For this review, take the finished solid that the model builds, in its own axes (mm). A direction names the side the tool comes from. Coordinates: 2 decimals unless noted, no trailing zeros. Loops run counter-clockwise (first coordinate to the right, second up) from the corner with the lowest first, then second, coordinate; pieces in that order, holes last. Notation, with made-up numbers: M 61,75.5 L 95,75.5 A29 ccw 95,107.5 Z; hole C -40,70.25 d2. An arc over 180 degrees is marked long. Put each result on its own line as item: value.
```python
from build123d import *

# Parameters (mm, degrees)
SKETCH_W        = 66
SKETCH_H        = 60
PAD_DEPTH       = 2
FILLET_R        = 4
SKETCH001_R     = 1.75
POCKET_DEPTH    = 2.001
PAD001_DEPTH    = 2
POCKET001_DEPTH = 2
FILLET001_R     = 1
FILLET002_R     = 1
FILLET003_R     = 1
FILLET004_R     = 1


with BuildPart() as part:
    # Sketch → Pad (new body)
    with BuildSketch(Plane.XY):
        Rectangle(SKETCH_W, SKETCH_H)
    extrude(amount=PAD_DEPTH)

    # Fillet
    fillet_edges = [part.edges().sort_by_distance(p)[0] for p in [
        (-33, -30, 1),
        (33, -30, 1),
        (33, 30, 1),
        (-33, 30, 1),
    ]]
    fillet(fillet_edges, radius=FILLET_R)

    # Sketch001 (on Face5 of Fillet) → Pocket (cut, through all)
    with BuildSketch(Plane.XY.offset(2)):
        with Locations((-29, 26)):
            Circle(SKETCH001_R)
        with Locations((29, 26)):
            Circle(SKETCH001_R)
        with Locations((29, -26)):
            Circle(SKETCH001_R)
        with Locations((-29, -26)):
            Circle(SKETCH001_R)
    extrude(amount=-POCKET_DEPTH, mode=Mode.SUBTRACT)

    # Sketch002 (on Face5 of Pocket) → Pad001 (join)
    with BuildSketch(Plane.XY.offset(2)):
        with BuildLine():
            ThreePointArc((-29.8, 22.901613), (-26.737258, 23.737258), (-25.901613, 26.8))
            Line((-25.901613, 26.8), (25.901613, 26.8))
            ThreePointArc((25.901613, 26.8), (26.737258, 23.737258), (29.8, 22.901613))
            Line((29.8, 22.901613), (29.8, -22.901613))
            ThreePointArc((29.8, -22.901613), (26.737258, -23.737258), (25.901613, -26.8))
            Line((-25.901613, -26.8), (25.901613, -26.8))
            ThreePointArc((-25.901613, -26.8), (-26.737258, -23.737258), (-29.8, -22.901613))
            Line((-29.8, 22.901613), (-29.8, -22.901613))
        make_face()
    extrude(amount=PAD001_DEPTH)

    # Sketch003 (on Face23 of Pad001) → Pocket001 (cut)
    with BuildSketch(Plane.XY.offset(4)):
        with BuildLine():
            ThreePointArc((-26.6, 20.283358), (-24.615938, 21.615938), (-23.283358, 23.6))
            Line((23.283358, 23.6), (-23.283358, 23.6))
            ThreePointArc((23.283358, 23.6), (24.615938, 21.615938), (26.6, 20.283358))
            Line((26.6, -20.283358), (26.6, 20.283358))
            ThreePointArc((26.6, -20.283358), (24.615938, -21.615938), (23.283358, -23.6))
            Line((-23.283358, -23.6), (23.283358, -23.6))
            ThreePointArc((-23.283358, -23.6), (-24.615938, -21.615938), (-26.6, -20.283358))
            Line((-26.6, 20.283358), (-26.6, -20.283358))
        make_face()
    extrude(amount=-POCKET001_DEPTH, mode=Mode.SUBTRACT)

    # Fillet001
    fillet001_edges = [part.edges().sort_by_distance(p)[0] for p in [
        (-25.901613, 26.8, 3),
        (-29.8, 22.901613, 3),
        (-29.8, -22.901613, 3),
        (-25.901613, -26.8, 3),
        (25.901613, 26.8, 3),
        (29.8, 22.901613, 3),
        (29.8, -22.901613, 3),
        (25.901613, -26.8, 3),
    ]]
    fillet(fillet001_edges, radius=FILLET001_R)

    # Fillet002
    fillet002_edges = [part.edges().sort_by_distance(p)[0] for p in [
        (-26.6, 20.283358, 3),
        (-23.283358, 23.6, 3),
        (23.283358, 23.6, 3),
        (26.6, 20.283358, 3),
        (26.6, -20.283358, 3),
        (23.283358, -23.6, 3),
        (-26.6, -20.283358, 3),
        (-23.283358, -23.6, 3),
    ]]
    fillet(fillet002_edges, radius=FILLET002_R)

    # Fillet003
    fillet003_edges = [part.edges().sort_by_distance(p)[0] for p in [
        (0, -23.6, 4),
        (-23.167049, -23.457969, 4),
        (23.167049, -23.457969, 4),
        (-24.615938, -21.615938, 4),
        (24.615938, -21.615938, 4),
        (-26.457969, -20.167049, 4),
        (26.457969, -20.167049, 4),
        (-26.6, 0, 4),
        (26.6, 0, 4),
        (-26.457969, 20.167049, 4),
        (26.457969, 20.167049, 4),
        (-24.615938, 21.615938, 4),
        (24.615938, 21.615938, 4),
        (-23.167049, 23.457969, 4),
        (23.167049, 23.457969, 4),
        (0, 23.6, 4),
        (-26.737258, -23.737258, 4),
        (-25.49483, -26.523747, 4),
        (-29.523747, -22.49483, 4),
        (0, -26.8, 4),
        (-29.8, 0, 4),
        (25.49483, -26.523747, 4),
        (-29.523747, 22.49483, 4),
        (26.737258, -23.737258, 4),
        (-26.737258, 23.737258, 4),
        (29.523747, -22.49483, 4),
        (-25.49483, 26.523747, 4),
        (29.8, 0, 4),
        (0, 26.8, 4),
        (29.523747, 22.49483, 4),
        (25.49483, 26.523747, 4),
        (26.737258, 23.737258, 4),
    ]]
    fillet(fillet003_edges, radius=FILLET003_R)

    # Fillet004
    fillet004_edges = [part.edges().sort_by_distance(p)[0] for p in [
        (0, -30, 0),
    ]]
    fillet(fillet004_edges, radius=FILLET004_R)


solid = part.part
```
(1) Add section A-A (y = -7.5). Write out the cut boundary in (x, z), plus the area to 3 significant figures.
Determined:
outline: M -33,1 A1 ccw -32,0 L 32,0 A1 ccw 33,1 L 33,2 L 29.8,2 L 29.8,3 A1 ccw 28.8,4 L 27.6,4 A1 ccw 26.6,3 L 26.6,2 L -26.6,2 L -26.6,3 A1 ccw -27.6,4 L -28.8,4 A1 ccw -29.8,3 L -29.8,2 L -33,2 Z
area: 144 mm^2
(2) For pin 1 (0.8 mm diameter, centred on y = -5, z = 2.5, fed in from -X); pin 2 (10 mm diameter, centred on x = 9.5, y = 3, fed in from +Z); pin 3 (0.8 mm diameter, centred on x = -6, z = 2.5, fed in from -Y), all flat-tipped, find the tip position at first contact; note any pin that passes through.
Determined:
pin 1: stops at x = -29.8
pin 2: stops at z = 2
pin 3: stops at y = -26.8
(3) Tool access review of faces 1 (the cylindrical face through (-26.761, 23.714, 2.493)), 2 (the flat face through (0, 0, 0)), 3 (the cylindrical face through (-24.6, -21.63, 2.51)), 4 (the cylindrical face through (26.714, 23.761, 2.493)), 5 (the cylindrical face through (-26.714, -23.761, 2.493)): name each direction out of +Z, -Z, +X, -X, +Y, -Y from which nothing blocks a thin tool from reaching the whole face with its end or side.
Determined:
face 1: +Z, -X, +Y
face 2: -Z, +X, -X, +Y, -Y
face 3: +Z
face 4: +Z, +X, +Y
face 5: +Z, -X, -Y
(4) Draft analysis for pull direction Y (two halves, no side actions). For faces 6 (the cylindrical face through (26.761, -23.714, 2.493)), 7 (the flat face through (0, 27, 2)), 8 (the cylindrical face through (-31.859, 28.797, 1.507)), 9 (the cylindrical face through (-24.63, 21.6, 2.51)), state which applies: +Y half, -Y half, draft (parallel to the pull), parting line (faces both ways), or undercut.
Determined:
face 6: -Y half
face 7: draft
face 8: +Y half
face 9: undercut
(5) Add section B-B (x = 5.5). Write out the cut boundary in (y, z), plus the area to 3 significant figures.
Determined:
outline: M -30,1 A1 ccw -29,0 L 29,0 A1 ccw 30,1 L 30,2 L 26.8,2 L 26.8,3 A1 ccw 25.8,4 L 24.6,4 A1 ccw 23.6,3 L 23.6,2 L -23.6,2 L -23.6,3 A1 ccw -24.6,4 L -25.8,4 A1 ccw -26.8,3 L -26.8,2 L -30,2 Z
area: 132 mm^2
(6) Wall thickness on line 1 along Y through (x, z) = (29, 1.4); line 2 along X through (y, z) = (16, 2.25); line 3 along Y through (x, z) = (-14.5, 2.25): over which ranges is each line inside the solid? List them lowest first. Write a range as [from, to].
Determined:
line 1: y = [-30, -27.75], [-24.25, 24.25], [27.75, 30]
line 2: x = [-29.8, -26.6], [26.6, 29.8]
line 3: y = [-26.8, -23.6], [23.6, 26.8]
